Answer from the drawing. Dimensions are ordinates in mm from the lowest x, y and z of the part. A direction names the side the tool comes from. Give positions to 0.01 mm unless a question says otherwise; leave off trailing zeros. Loops run counter-clockwise (first coordinate to the right, second up) from the corner with the lowest first, then second, coordinate; pieces in that order, holes last.
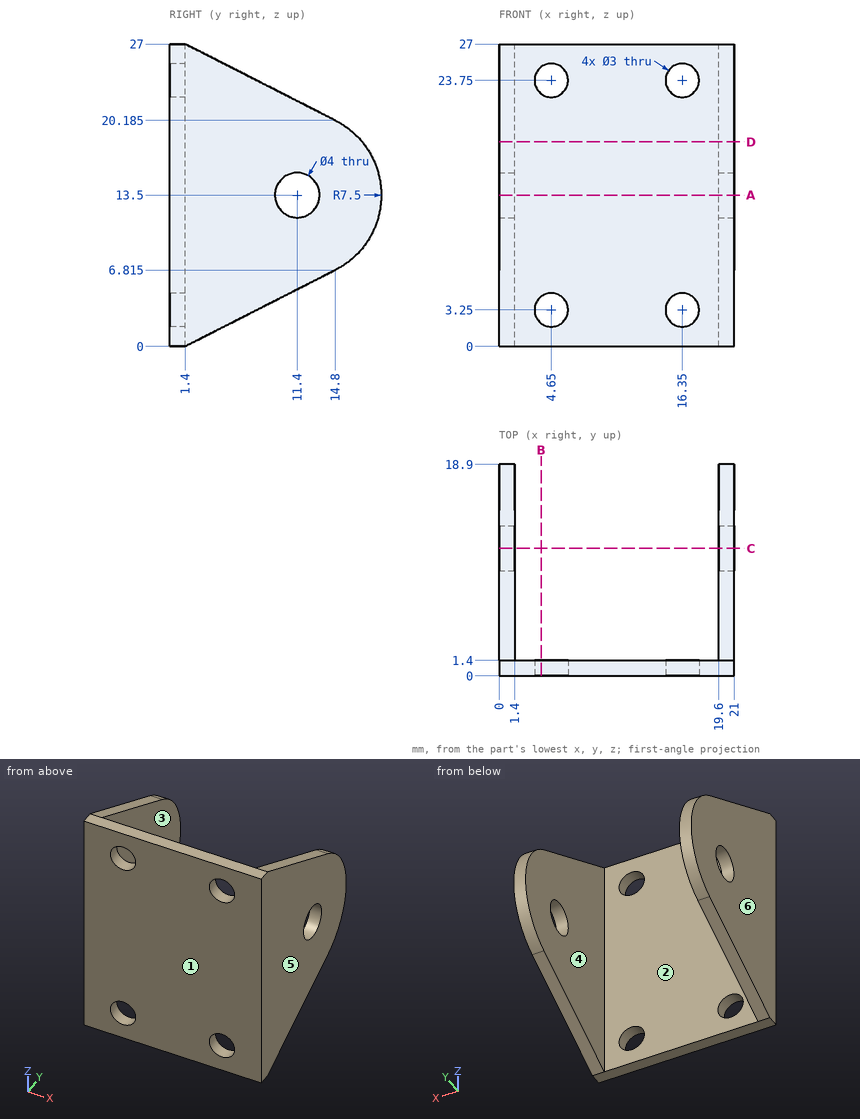
Item 1: Determine the mould class of the marked faces 3, 4, 5 and 6 for opening direction X: released by +X, released by -X, zero draft, split by the parting line, or undercut.
Item 2: For the marked faces 1 and 2, determine the directions among +Z, -Z, +X, -X, +Y, -Y from which every point of the face is accessible in a straight line to the end or side of a thin tool.
Item 3: Find section D-D, the plane z = 18.25. Write down the section's boundary in (x, y).
Item 4: Consider line 1 (X direction, y = 0.75, z = 3.25); line 2 (Z direction, x = 16.35, y = 0.9); line 3 (X direction, y = 5.25, z = 24). Determine where each line is inside the solid, lowest interval first.
Item 5: Find section C-C, the plane y = 11.4. Write down the section's boundary in (x, z).
Item 6: Find section B-B, the plane x = 3.75. Write down the section's boundary in (y, z).
Item 7: Flat-ended cylindrical pins translate along their axes: pin 1 Ø4 at (x, z) = (2.5, 21) entering from +Y; pin 2 Ø3.5 at (x, z) = (16.35, 23.75) entering from +Y. Find the tip coordinate at first contact, or state that the pin passes through.
Item 8: Find section A-A, the plane z = 13.5. Write down the section's boundary in (x, y).
Ans:
1. face 3: undercut
1. face 4: undercut
1. face 5: released by +X
1. face 6: released by -X
2. face 1: +Z, -Z, +X, -X, -Y
2. face 2: +Z, -Z, +Y
3. outline: (0, 0) - (21, 0) - (21, 17.2) - (19.6, 17.2) - (19.6, 1.4) - (1.4, 1.4) - (1.4, 17.2) - (0, 17.2) - close
4. line 1: x = 0 to 3.15, 6.15 to 14.85, 17.85 to 21
4. line 2: z = 0 to 1.75, 4.75 to 22.25, 25.25 to 27
4. line 3: x = 0 to 1.4, 19.6 to 21
5. outline: (0, 5.09) - (1.4, 5.09) - (1.4, 11.5) - (0, 11.5) - close; (0, 15.5) - (1.4, 15.5) - (1.4, 21.91) - (0, 21.91) - close; (19.6, 5.09) - (21, 5.09) - (21, 11.5) - (19.6, 11.5) - close; (19.6, 15.5) - (21, 15.5) - (21, 21.91) - (19.6, 21.91) - close
6. outline: (0, 0) - (1.4, 0) - (1.4, 2.05) - (0, 2.05) - close; (0, 4.45) - (1.4, 4.45) - (1.4, 22.55) - (0, 22.55) - close; (0, 24.95) - (1.4, 24.95) - (1.4, 27) - (0, 27) - close
7. pin 1: stops at y = 16.12
7. pin 2: stops at y = 1.4
8. outline: (0, 0) - (21, 0) - (21, 9.4) - (19.6, 9.4) - (19.6, 1.4) - (1.4, 1.4) - (1.4, 9.4) - (0, 9.4) - close; (0, 13.4) - (1.4, 13.4) - (1.4, 18.9) - (0, 18.9) - close; (19.6, 13.4) - (21, 13.4) - (21, 18.9) - (19.6, 18.9) - close
